```python
from build123d import *

# Parameters (mm, degrees)
ESQUISSE1_W        = 60
ESQUISSE1_H        = 46
ESQUISSE1_W_2      = 12
ESQUISSE1_H_2      = 30
BOSS_EXTRU_1_DEPTH = 5


with BuildPart() as part:
    # Esquisse1 → Boss.-Extru.1 (new body)
    # profile 1 of 2: a face of its own
    with BuildSketch(Plane.XY):
        with Locations((-3.893592945, 15.1875)):
            Rectangle(ESQUISSE1_W, ESQUISSE1_H)
        Polygon((-14.893592945, 25.1875), (-9.893592945, 25.1875), (-9.893592945, 30.1875), (2.106407055, 30.1875), (2.106407055, 25.1875), (7.106407055, 25.1875), (7.106407055, 20.1875), (2.106407055, 20.1875), (2.106407055, 10.1875), (7.106407055, 10.1875), (7.106407055, 5.1875), (2.106407055, 5.1875), (2.106407055, 0.1875), (-9.893592945, 0.1875), (-9.893592945, 5.1875), (-14.893592945, 5.1875), (-14.893592945, 10.1875), (-9.893592945, 10.1875), (-9.893592945, 20.1875), (-14.893592945, 20.1875), align=None, mode=Mode.SUBTRACT)
    # profile 2 of 2: a face of its own
    with BuildSketch(Plane.XY):
        with Locations((-3.893592945, 15.1875)):
            Rectangle(ESQUISSE1_W_2, ESQUISSE1_H_2)
    extrude(amount=BOSS_EXTRU_1_DEPTH)


solid = part.part
```
Check sheet for the modelled part. Datum: model origin and axes. Units: mm. A direction names the side the tool comes from. Round coordinates to 2 decimals unless told otherwise and drop trailing zeros. Loops run counter-clockwise (first coordinate to the right, second up) from the corner with the lowest first, then second, coordinate; pieces in that order, holes last. Notation, with made-up numbers: (82, 34.5) - (90, 34.5) arc R18 cw to (90, 60.5) - close; hole circle Ø4 at (45.5, 77). An arc over 180 degrees is marked (long way). Write item = value, one per line. Start each with the question number.
Q1. Access from +Z, -Z, +X, -X, +Y, -Y to the whole of each face (thin tool, end or side, straight path). Record for faces 5 (the face through (-4, 16, 5)), 6 (the face through (-14.894, 8, 2)).
Q2. Release check for a two-part mould opening along X. For faces 1 (the face through (26.106, 15, 2)), 2 (the face through (-4, -7.812, 2)), 3 (the face through (-9.894, 8, 2)), 4 (the face through (-33.894, 15, 2)) record: pulls with the +X half, pulls with the -X half, needs draft (parallel to the pull), parting line crosses it, or undercut.
Q3. Section check B-B (y = 7). Record the boundary of the cut face in (x, z).
Q4. Thickness scan on L1, parallel to X at y = 8, z = 4.6; L2, parallel to Y at x = 6, z = 2.7. Record the ranges inside material, lowest first.
Q5. Section check A-A (z = 3.9). Record the boundary of the cut face in (x, y), plus the area to 3 significant figures.
Derived:
q1.face_5 = +Z, +X, -X, +Y, -Y
q1.face_6 = +Z, -Z
q2.face_1 = pulls with the +X half
q2.face_2 = needs draft
q2.face_3 = undercut
q2.face_4 = pulls with the -X half
q3.outline = (-33.89, 0) - (-14.89, 0) - (-14.89, 5) - (-33.89, 5) - close; (-9.89, 0) - (2.11, 0) - (2.11, 5) - (-9.89, 5) - close; (7.11, 0) - (26.11, 0) - (26.11, 5) - (7.11, 5) - close
q4.L1 = -33.89 to -14.89, -9.89 to 2.11, 7.11 to 26.11
q4.L2 = -7.81 to 5.19, 10.19 to 20.19, 25.19 to 38.19
q5.outline = (-33.89, -7.81) - (26.11, -7.81) - (26.11, 38.19) - (-33.89, 38.19) - close; hole (-14.89, 5.19) - (-9.89, 5.19) - (-9.89, 10.19) - (-14.89, 10.19) - close; hole (-14.89, 20.19) - (-9.89, 20.19) - (-9.89, 25.19) - (-14.89, 25.19) - close; hole (2.11, 5.19) - (7.11, 5.19) - (7.11, 10.19) - (2.11, 10.19) - close; hole (2.11, 20.19) - (7.11, 20.19) - (7.11, 25.19) - (2.11, 25.19) - close
q5.area = 2,660 mm^2
